from build123d import *

# Parameters (mm, degrees)
SKETCH1_R           = 15
BOSS_EXTRUDE1_DEPTH = 35
SKETCH2_OUTSIDE_W   = 110.904
SKETCH2_OUTSIDE_H   = 101.622
SKETCH2_OUTSIDE_R   = 30
CUT_EXTRUDE1_DEPTH  = 10
CUT_EXTRUDE1_TAPER  = 45


with BuildPart() as part:
    # Sketch1 → Boss-Extrude1 (new body)
    with BuildSketch(Plane(origin=(0, 0, 0), x_dir=(1, 0, 0), z_dir=(0, 1, 0))):
        Polygon((34.641016151, 0), (17.320508076, 30), (-17.320508076, 30), (-34.641016151, 0), (-17.320508076, -30), (17.320508076, -30), align=None)
        Circle(SKETCH1_R, mode=Mode.SUBTRACT)
    extrude(amount=BOSS_EXTRUDE1_DEPTH)

    # Sketch2 outside → Cut-Extrude1 (cut)
    with BuildSketch(Plane(origin=(0, 35, 0), x_dir=(1, 0, 0), z_dir=(0, 1, 0))):
        Rectangle(SKETCH2_OUTSIDE_W, SKETCH2_OUTSIDE_H)
        Circle(SKETCH2_OUTSIDE_R, mode=Mode.SUBTRACT)
    extrude(amount=-CUT_EXTRUDE1_DEPTH, taper=CUT_EXTRUDE1_TAPER, mode=Mode.SUBTRACT)


solid = part.part
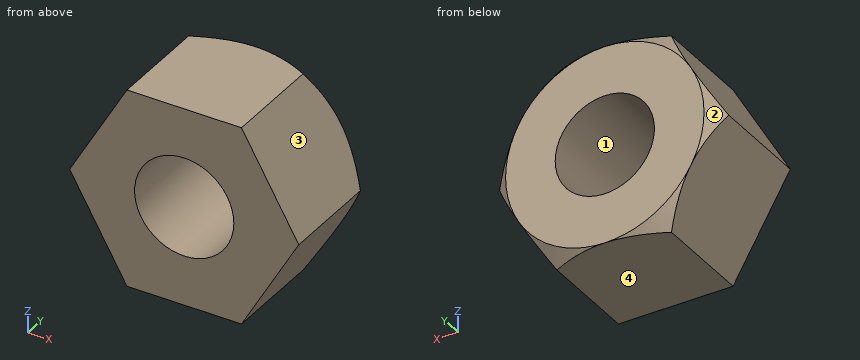
Can you work these out from the model? Positions are in its coordinate system, mm. Face numbers are marked on the shaded views. Give positions to 0.01 mm unless a question says otherwise; leave off trailing zeros. Write each loop counter-clockwise with the first axis right and the second up, starting at its lowest first coordinate (ties: lowest second). Pieces come first, ordered by that corner, then holes. Notation, with made-up numbers: (16, 81) -> (32, 81) arc R32 ccw to (32, 116) -> close; hole circle Ø11 at (-17.75, 29). An arc over 180 degrees is marked (long way). Answer as a JSON object with one key per item and string values. Group by question number.
Item 1: Suppose I cut it at A-A (y = 25). Please give me the cut outline in (x, z), plus the area to 3 significant figures.
Item 2: We'd pull the mould along Z, two halves only. Please class the marked faces 1, 2, 3 and 4: +Z half, -Z half, draft (parallel to the pull), parting line (faces both ways), or undercut.
Item 3: I'm going to push flat-ended pins straight in: P1, Ø1.5, axis at y = 18.5, z = -16.5, coming from the +X side; P2, Ø12, axis at y = 20, z = 7.5, coming from the -X side (3 decimals); P3, Ø6, axis at x = -22.5, y = 10.5, coming from the -Z side (3 decimals); P4, Ø3, axis at x = 0.5, z = 23.5, coming from the -Y side. Where does each tip first touch, or does it pass through?
Item 4: Please list where these lines run through material, in increasing order: line 1 (Z direction, x = 0, y = 18); line 2 (X direction, y = 22, z = 0); line 3 (Z direction, x = 10.5, y = 33). Write a range as [from, to].
Findings:
{
 "1": {"outline": "(-34.64, 0) -> (-17.32, -30) -> (17.32, -30) -> (34.64, 0) -> (17.32, 30) -> (-17.32, 30) -> close; hole circle Ø30 at (0, 0)", "area": "2,410 mm²"},
 "2": {"face 1": "undercut", "face 2": "parting line", "face 3": "+Z half", "face 4": "-Z half"},
 "3": {"P1": "stops at x = 25.55", "P2": "stops at x = -33.775", "P3": "stops at z = -26.225", "P4": "stops at y = 0"},
 "4": {"line 1": "z = [-30, -15], [15, 30]", "line 2": "x = [-34.64, -15], [15, 34.64]", "line 3": "z = [-30, -10.71], [10.71, 30]"}
}
